For this review, take the finished solid that the model builds, in its own axes (mm). Face numbers are marked on the shaded views. Coordinates: 2 decimals unless noted, no trailing zeros. Order: outer loops, then holes, each group sorted by start corner. A loop starts at its lowest first (then second) coordinate and runs counter-clockwise, first axis right, second up. Notation, with made-up numbers: M 88,63.25 L 131,63.25 A11 ccw 131,70.25 Z; hole C 32,76.5 d3. An arc over 180 degrees is marked long. Use CSV: the item, a comma, the result in double quotes.
```python
from build123d import *

# Parameters (mm, degrees)
SKETCH1_R           = 7.5
BOSS_EXTRUDE2_DEPTH = 20


with BuildPart() as part:
    # Sketch1 → Boss-Extrude2 (new body)
    # profile 1 of 5: a face of its own
    with BuildSketch(Plane.XY):
        with BuildLine():
            ThreePointArc((7.5, 10), (6.696925103, 4.759514134), (4.361406616, 0))
            Line((4.361406616, 0), (115.638593384, 0))
            ThreePointArc((115.638593384, 0), (112.5, 10), (115.638593384, 20))
            Line((115.638593384, 20), (4.361406616, 20))
            ThreePointArc((4.361406616, 20), (6.696925103, 15.240485866), (7.5, 10))
        make_face()
    # profile 2 of 5: a face of its own
    with BuildSketch(Plane.XY):
        with BuildLine():
            Line((0, 20), (0, 0))
            Line((0, 0), (4.361406616, 0))
            ThreePointArc((4.361406616, 0), (6.696925103, 4.759514134), (7.5, 10))
            ThreePointArc((7.5, 10), (6.696925103, 15.240485866), (4.361406616, 20))
            Line((4.361406616, 20), (0, 20))
        make_face()
    # profile 3 of 5: a face of its own
    with BuildSketch(Plane.XY):
        with BuildLine():
            ThreePointArc((115.638593384, 20), (112.5, 10), (115.638593384, 0))
            Line((115.638593384, 0), (120, 0))
            Line((120, 0), (120, 20))
            Line((120, 20), (115.638593384, 20))
        make_face()
    # profile 4 of 5: a face of its own
    with BuildSketch(Plane.XY):
        with BuildLine():
            Line((120, 0), (115.638593384, 0))
            ThreePointArc((115.638593384, 0), (135.240485866, -6.696925103), (147.5, 10))
            ThreePointArc((147.5, 10), (135.240485866, 26.696925103), (115.638593384, 20))
            Line((115.638593384, 20), (120, 20))
            Line((120, 20), (120, 0))
        make_face()
        with Locations((130, 10)):
            Circle(SKETCH1_R, mode=Mode.SUBTRACT)
    # profile 5 of 5: a face of its own
    with BuildSketch(Plane.XY):
        with BuildLine():
            Line((4.361406616, 0), (0, 0))
            Line((0, 0), (0, 20))
            Line((0, 20), (4.361406616, 20))
            ThreePointArc((4.361406616, 20), (-27.5, 10), (4.361406616, 0))
        make_face()
        with Locations((-10, 10)):
            Circle(SKETCH1_R, mode=Mode.SUBTRACT)
    extrude(amount=BOSS_EXTRUDE2_DEPTH)


solid = part.part
```
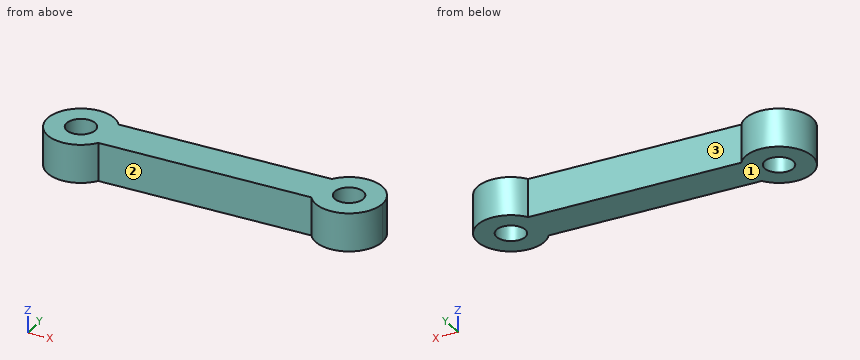
Item 1: Clearance check with flat-ended pins moving along their axes: pin 1 Ø12 at (y, z) = (18.5, 15) entering from +X; pin 2 Ø2 at (y, z) = (-3, 7) entering from +X; pin 3 Ø1.5 at (x, z) = (76.5, 11.5) entering from +Y. State where each tip first meets the part, or that it passes through.
Solutions:
pin 1,"x = 147.32"
pin 2,"x = 142.74"
pin 3,"y = 20"
Item 2: Draft analysis for pull direction X (two halves, no side actions). For the marked faces 1, 2 and 3, state which applies: released by +X, released by -X, zero draft, split by the parting line, or undercut.
Solutions:
face 1,"zero draft"
face 2,"undercut"
face 3,"undercut"
Item 3: Add section C-C on y = -4. State the section outline as (x, z) points.
Solutions:
outline,"M -20.5,0 L 0.5,0 L 0.5,20 L -20.5,20 Z; M 119.5,0 L 140.5,0 L 140.5,20 L 119.5,20 Z"
Item 4: To check wall thickness, follow line 1 along Y through (x, z) = (-10, 13.25); line 2 along X through (y, z) = (5, 17.25); line 3 along Y through (x, z) = (114, 4). State the ranges of each line that lie inside material, in increasing order. Write a range as [from, to].
Solutions:
line 1,"[-7.5, 2.5], [17.5, 27.5]"
line 2,"[-26.77, -15.59], [-4.41, 124.41], [135.59, 146.77]"
line 3,"[0, 20]"
Item 5: Add section B-B on z = 5. State the section outline as (x, y) points, and give its area (3 significant figures).
Solutions:
outline,"M 4.36,0 L 115.64,0 A17.5 ccw long 115.64,20 L 4.36,20 A17.5 ccw long Z; hole C -10,10 d15; hole C 130,10 d15"
area,"3,710 mm^2"
Item 6: Add section D-D on y = 4. State the section outline as (x, z) points.
Solutions:
outline,"M -26.44,0 L -14.5,0 L -14.5,20 L -26.44,20 Z; M -5.5,0 L 125.5,0 L 125.5,20 L -5.5,20 Z; M 134.5,0 L 146.44,0 L 146.44,20 L 134.5,20 Z"
Item 7: Add section A-A on x = 130. State the section outline as (y, z) points.
Solutions:
outline,"M -7.5,0 L 2.5,0 L 2.5,20 L -7.5,20 Z; M 17.5,0 L 27.5,0 L 27.5,20 L 17.5,20 Z"
